The figure shows three views and two pictorial views of one solid part (mm, origin at its lowest corner). Answer the questions. A direction names the side the tool comes from. Round coordinates to 2 decimals unless told otherwise and drop trailing zeros. Write each loop counter-clockwise with the first axis right and the second up, starting at its lowest first coordinate (ties: lowest second). Pieces come first, ordered by that corner, then holes. Notation, with made-up numbers: (76, -26.5) -> (134, -26.5) arc R26 ccw to (134, -4.5) -> close; hole circle Ø6 at (-35, -14.5). An arc over 180 degrees is marked (long way). One line per item, written item: value.
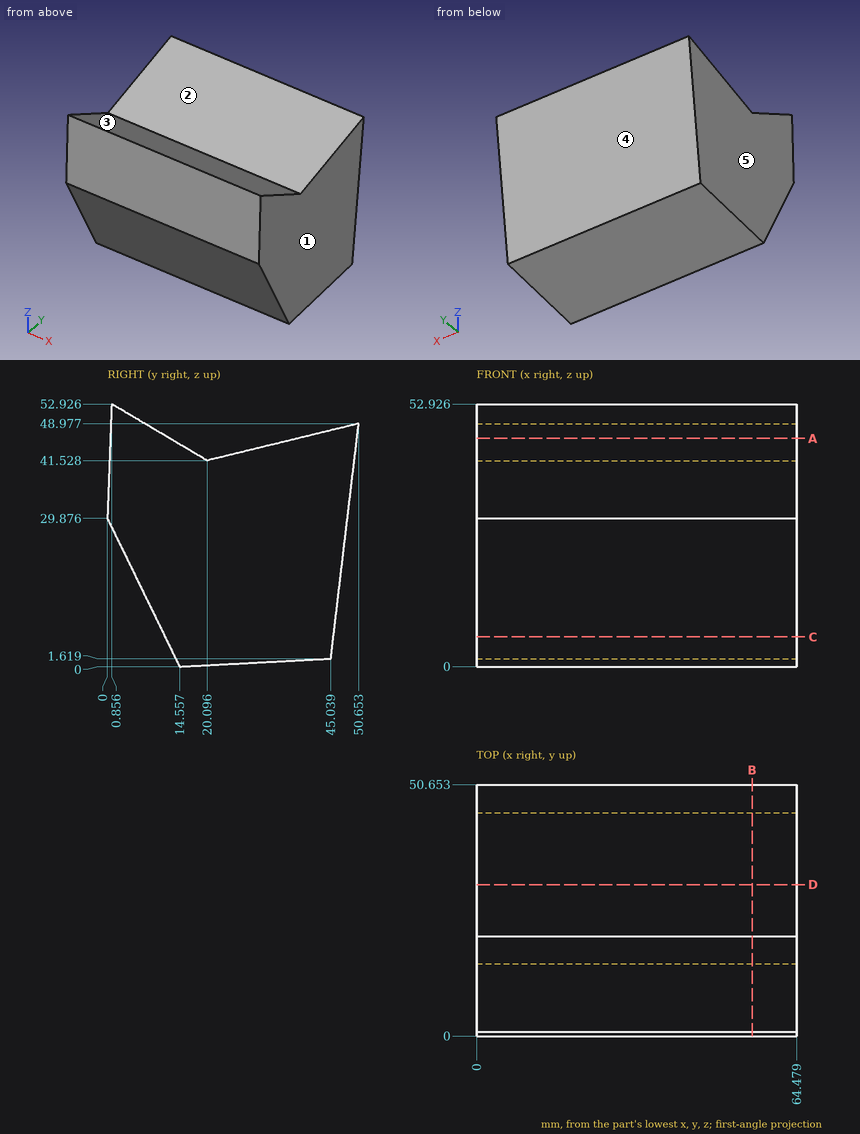
(1) For a pull along Y with two mould halves and no side action, classify the marked faces 3, 4 and 5 as pulls with the +Y half, pulls with the -Y half, needs draft (parallel to the pull), parting line crosses it, or undercut.
Reported:
face 3: undercut
face 4: pulls with the +Y half
face 5: needs draft
(2) A tool of negligible diameter and unlimited length cuts with its end or side. For the marked faces 1 and 2, from which of +Z, -Z, +X, -X, +Y, -Y can it reach the whole face along a straight path? Write none if from no direction.
Reported:
face 1: +Z, -Z, +X, +Y, -Y
face 2: +Z, +X, -X
(3) Find section C-C on z = 6. Give the vertices of the cut face in (x, y).
Reported:
outline: (0, 11.63) -> (64.48, 11.63) -> (64.48, 45.56) -> (0, 45.56) -> close
(4) Consider probe 1 along Y at (x, z) = (29, 33) (1 decimal); probe 2 along Y at (x, z) = (3, 5); probe 3 along Z at (x, y) = (59, 20.5) (1 decimal). Determine where each line is inside the solid, lowest interval first.
Reported:
probe 1: y = 0.1 to 48.8
probe 2: y = 12.12 to 45.44
probe 3: z = 0.3 to 41.6
(5) Find section B-B on x = 55.5. Give the vertices of the cut face in (y, z) (1 decimal).
Reported:
outline: (0, 29.9) -> (14.6, 0) -> (45, 1.6) -> (50.7, 49) -> (20.1, 41.5) -> (0.9, 52.9) -> close
(6) Find section D-D on y = 30.5. Give the vertices of the cut face in (x, z).
Reported:
outline: (0, 0.85) -> (64.48, 0.85) -> (64.48, 44.06) -> (0, 44.06) -> close
(7) Flat-ended cylindrical pins translate along their axes: pin 1 Ø3 at (y, z) = (31.5, 36.5) entering from -X; pin 2 Ø4 at (x, y) = (53, 23) entering from -Z; pin 3 Ø6 at (x, z) = (38, 13.5) entering from -Y; pin 4 Ø1.5 at (x, z) = (56.5, 42) entering from -Y. Find the tip coordinate at first contact, or state that the pin passes through.
Reported:
pin 1: stops at x = 0
pin 2: stops at z = 0.34
pin 3: stops at y = 6.52
pin 4: stops at y = 0.42
(8) Find section A-A on z = 46. Give the vertices of the cut face in (x, y), plus the area to 4 significant figures.
Reported:
outline: (0, 0.6) -> (64.48, 0.6) -> (64.48, 12.55) -> (0, 12.55) -> close; (0, 38.44) -> (64.48, 38.44) -> (64.48, 50.3) -> (0, 50.3) -> close
area: 1,535 mm2
